The listing builds one solid part. Answer for the finished solid, in the listing's coordinates (mm). A direction names the side the tool comes from. Give positions to 0.01 mm unless a question says otherwise; leave off trailing zeros. Write each loop counter-clockwise with the first axis right and the second up, starting at its lowest first coordinate (ties: lowest second). Pieces come first, ordered by that corner, then holes. Notation, with made-up numbers: (65.5, 7.25) - (112.5, 7.25) arc R29 ccw to (112.5, 30.25) - close; hole circle Ø3 at (56, 62). An arc over 180 degrees is marked (long way). Answer as CSV lines item,"result". Start each with the question number.
(1) Each of these flat-tipped pins is pushed along its axis until it touches: pin 1 Ø14.5 at (x, y) = (8, 7.5) entering from +Z; pin 2 Ø6 at (y, z) = (28.5, 32) entering from +X; pin 3 Ø7.5 at (x, z) = (19, 21.5) entering from -Y. Where does it stop, or does it pass through?
(2) Find section A-A (z = 18). Write down the section's boundary in (x, y), then the cut area to 3 significant figures.
(3) For a pull along Y with two mould halves and no side action, classify faces 1 (the face through (-33, 29.029, 25)), 2 (the face through (-35.611, 9.836, 6.261)), 3 (the face through (-51.09, 15, 6)) as pulls with the +Y half, pulls with the -Y half, needs draft (parallel to the pull), parting line crosses it, or undercut.
(4) Find section B-B (y = 20). Write down the section's boundary in (x, z).
(5) For faces 4 (the face through (34.639, 34, 13)), 5 (the face through (-14.583, 18, 22)), 6 (the face through (-4.62, 18, 22)), 7 (the face through (-51.09, 34, 13)), determine the directions among +Z, -Z, +X, -X, +Y, -Y from which every point of the face is accessible in a straight line to the end or side of a thin tool.
(6) Find section C-C (x = 4.5). Write down the section's boundary in (y, z), then the cut area to 3 significant figures.
(7) Straight lines are drawn through the part: probe 1 along X at (y, z) = (19.5, 7); probe 2 along Z at (x, y) = (17, 3.5); probe 3 along Y at (x, z) = (21, 17.5). For each, find the intervals that lie inside material, in ascending order.
(8) Find section D-D (y = 30.5). Write down the section's boundary in (x, z).
from build123d import *

# Parameters (mm, degrees)
F0_R     = 10.182819
F0_R_2   = 10.195674
F0_W     = 85.729957
F0_H     = 9.931274
F1_DEPTH = 12.7
F2_W     = 85.729957
F2_H     = 9.931274
F3_DEPTH = 25.4
F4_SIZE  = 12.7
F5_SIZE  = 12.7
F6_W     = 9.963379
F6_H     = 29.028814
F7_DEPTH = 25.4
F8_SIZE  = 25.4


with BuildPart() as f1:
    # F0 (on Top) → F1 (new body)
    with BuildSketch(Plane.XY):
        Polygon((-51.090479, 0), (34.932677, 0), (34.932677, 29.028814), (34.639478, 29.028814), (-51.090479, 29.028814), align=None)
        with Locations((-27.52999, 16.03223)):
            Circle(F0_R, mode=Mode.SUBTRACT)
        with Locations((10.635439, 15.799049)):
            Circle(F0_R_2, mode=Mode.SUBTRACT)
        with Locations((-8.2255, 33.994451)):
            Rectangle(F0_W, F0_H)
    extrude(amount=F1_DEPTH)

    # F2 (on face) → F3 (join)
    with BuildSketch(Plane.XY.offset(12.7)):
        with Locations((-8.2255, 33.994451)):
            Rectangle(F2_W, F2_H)
    extrude(amount=F3_DEPTH)

    # F4
    f4_edges = [f1.edges().sort_by_distance(p)[0] for p in [
        (34.639478, 33.994451, 38.1),
    ]]
    chamfer(f4_edges, length=F4_SIZE)

    # F5
    f5_edges = [f1.edges().sort_by_distance(p)[0] for p in [
        (-51.090479, 33.994451, 38.1),
    ]]
    chamfer(f5_edges, length=F5_SIZE)

    # F6 (on face) → F7 (join)
    with BuildSketch(Plane.XY.offset(12.7)):
        with Locations((-9.60124, 14.514407)):
            Rectangle(F6_W, F6_H)
    extrude(amount=F7_DEPTH)

    # F8
    f8_edges = [f1.edges().sort_by_distance(p)[0] for p in [
        (-9.601241, 0, 38.1),
    ]]
    chamfer(f8_edges, length=F8_SIZE)


solid = f1.part
Result set:
1,pin 1,"z = 12.7"
1,pin 2,"x = 30.99"
1,pin 3,"y = 29.03"
2,outline,"(-51.09, 29.03) - (-14.58, 29.03) - (-14.58, 5.3) - (-4.62, 5.3) - (-4.62, 29.03) - (34.64, 29.03) - (34.64, 38.96) - (-51.09, 38.96) - close"
2,area,"1,090 mm^2"
3,face 1,"pulls with the -Y half"
3,face 2,"undercut"
3,face 3,"needs draft"
4,outline,"(-51.09, 0) - (-36.91, 0) - (-36.91, 12.7) - (-51.09, 12.7) - close; (-18.15, 0) - (1.35, 0) - (1.35, 12.7) - (-4.62, 12.7) - (-4.62, 32.7) - (-14.58, 32.7) - (-14.58, 12.7) - (-18.15, 12.7) - close; (19.93, 0) - (34.93, 0) - (34.93, 12.7) - (19.93, 12.7) - close"
5,face 4,"+Z, -Z, +X, +Y"
5,face 5,"+Z, -X, -Y"
5,face 6,"+Z, +X, -Y"
5,face 7,"+Z, -Z, -X, +Y, -Y"
6,outline,"(0, 0) - (7.66, 0) - (7.66, 12.7) - (0, 12.7) - close; (23.94, 0) - (38.96, 0) - (38.96, 38.1) - (29.03, 38.1) - (29.03, 12.7) - (23.94, 12.7) - close"
6,area,"540 mm^2"
7,probe 1,"-51.09 to -37.1, -17.96 to 1.14, 20.14 to 34.93"
7,probe 2,"0 to 12.7"
7,probe 3,"29.03 to 38.96"
8,outline,"(-51.09, 0) - (34.64, 0) - (34.64, 25.4) - (21.94, 38.1) - (-38.39, 38.1) - (-51.09, 25.4) - close"
